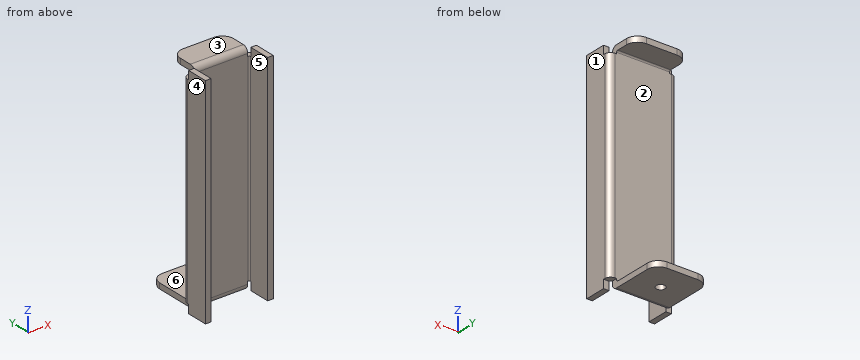
Autodesk Inventor part; units mm, degrees
ref_plane "YZ Plane" through (0, 0, 0) normal (1, 0, 0) x (0, 1, 0)
ref_plane "XZ Plane" through (0, 0, 0) normal (0, 1, 0) x (-1, 0, 0)
ref_plane "XY Plane" through (0, 0, 0) normal (0, 0, 1) x (1, 0, 0)
sketch "Эскиз1" plane through (0, 0, 0) normal (0, 0, 1) x (1, 0, 0)
  line L0 (0, 0) -> (0, 11.2754) construction
  line L1 (0, 0) -> (-17.0842, 0) construction
  line L2 (-12.15, 0) -> (12.15, 0)
  line L3 (12.15, 0) -> (12.15, 10.3)
  line L4 (12.15, 10.3) -> (-12.15, 10.3)
  line L5 (-12.15, 10.3) -> (-12.15, 0)
  line L6 (-10.15, 0) -> (10.15, 0)
  line L7 (10.15, 0) -> (10.15, 8.3)
  line L8 (10.15, 8.3) -> (-10.15, 8.3)
  line L9 (-10.15, 8.3) -> (-10.15, 0)
  dimension "d0" = 2
  dimension "d1" = 2
  dimension "d2" = 2
  dimension "d3" = 24.3
  dimension "d4" = 10.3
extrude "Выдавливание1" add sketch "Эскиз1" along normal mid plane 78 contours L5 L4 L3 L2 L7 L8 L9
sketch "Эскиз2" plane through (-12.15, 10.3, -39) normal (0, 1, 0) x (1, 0, 0)
  line L0 (0, 0) -> (24.3, 0)
  line L1 (2.65, 0) -> (21.65, 0)
  line L2 (21.65, 0) -> (21.65, -2)
  line L3 (21.65, -2) -> (2.65, -2)
  line L4 (2.65, -2) -> (2.65, 0)
  line L5 (24.3, -78) -> (0, -78)
  line L6 (2.65, -78) -> (21.65, -78)
  line L7 (21.65, -78) -> (21.65, -76)
  line L8 (21.65, -76) -> (2.65, -76)
  line L9 (2.65, -76) -> (2.65, -78)
  line L10 (12.15, -39) -> (12.15, -67.9082) construction
  dimension "d7" = 2
  dimension "d8" = 2
  dimension "d9" = 19
  dimension "d10" = 19
extrude "Выдавливание2" add sketch "Эскиз2" along normal blind 8.5 contours L5 L9 L8 L7
extrude "Выдавливание3" add sketch "Эскиз2" along normal blind 18 contours L0 L2 L3 L4
fillet "Сопряжение1" radius 4 4 edges at (9.5, 28.3, -38) (-9.5, 28.3, -38) (-9.5, 18.8, 38) (9.5, 18.8, 38)
sketch "Эскиз3" plane through (-9.5, 10.3, -37) normal (0, 0, 1) x (1, 0, 0)
  line L0 (9.5, -10.3) -> (9.5, 21.9843) construction
  circle A0 centre (9.5, 8) radius 1.6
  line L1 (15, 18) -> (4, 18)
  dimension "d16" = 3.2
  dimension "d17" = 10
extrude "Выдавливание4" cut sketch "Эскиз3" against normal blind 18
sketch "Эскиз4" plane through (0, 0, 39) normal (0, 0, 1) x (1, 0, 0)
  line L0 (12.15, 0) -> (12.15, 10.3)
  line L1 (9.5, 10.3) -> (12.15, 10.3)
  line L2 (12.15, 10.3) -> (12.15, 7.7)
  line L3 (12.15, 7.7) -> (9.5, 7.7)
  line L4 (9.5, 7.7) -> (9.5, 10.3)
  line L5 (10.15, 0) -> (12.15, 0)
  line L6 (-12.15, 10.3) -> (-9.5, 10.3)
  line L7 (-9.5, 10.3) -> (-15.4416, 10.3)
  line L8 (-15.4416, 10.3) -> (-15.4416, 7.7)
  line L9 (-15.4416, 7.7) -> (-9.5, 7.7)
  line L10 (-9.5, 7.7) -> (-9.5, 10.3)
  line L11 (-12.15, 0) -> (-10.15, 0)
  point P0 (0, 0)
  dimension "d20" = 7.7
  dimension "d21" = 7.7
extrude "Выдавливание5" cut sketch "Эскиз4" against normal blind 3
mirror "Зеркальное отражение1" about plane through (0, 0, 0) normal (0, 0, 1) of "Выдавливание5"
fillet "Сопряжение2" radius 2 4 edges at (0, 8.3, 39) (12.15, 10.3, 0) (-12.15, 10.3, 0) (0, 8.3, -39)
fillet "Сопряжение3" radius 0.5 4 edges at (0, 10.3, -37) (0, 10.3, 37) (10.15, 8.3, 0) (-10.15, 8.3, 0)
properties part number "крепление бабины"
CAD build for the part. Positions are in the model's coordinates, mm. Face numbers are marked on the shaded views. A direction names the side the tool comes from. Give positions to 0.01 mm unless a question says otherwise; leave off trailing zeros. Write each loop counter-clockwise with the first axis right and the second up, starting at its lowest first coordinate (ties: lowest second). Pieces come first, ordered by that corner, then holes. Notation, with made-up numbers: (-37, -12.75) -> (-16, -12.75) arc R17 cw to (-16, 11.25) -> close; hole circle Ø1 at (71.25, 43.25). An arc over 180 degrees is marked (long way). Return JSON: item names as keys, results as strings.
Item 1: Band-saw the part on B-B (x = 0). List the corners of the cut face in (y, z), then the cut area to 3 significant figures.
Answer below:
{"outline": "(8.3, -37) arc R2 ccw to (10.3, -39) -> (16.7, -39) -> (16.7, -37) -> (10.8, -37) arc R0.5 cw to (10.3, -36.5) -> (10.3, 36.5) arc R0.5 cw to (10.8, 37) -> (18.8, 37) -> (18.8, 39) -> (10.3, 39) arc R2 ccw to (8.3, 37) -> close; (19.9, -39) -> (28.3, -39) -> (28.3, -37) -> (19.9, -37) -> close", "area": "201 mm2"}
Item 2: Drop flat-ended pins along their axis: pin 1 (8 mm diameter, centred on x = -5, z = 15, fed in from -Y); pin 2 (1.6 mm diameter, centred on x = 11.5, z = 38, fed in from +Y); pin 3 (12 mm diameter, centred on y = 12.5, z = -19, fed in from -X); pin 4 (1.5 mm diameter, centred on y = 10, z = 37, fed in from -X). Give the stop position or say it passes through.
Answer below:
{"pin 1": "stops at y = 8.3", "pin 2": "stops at y = 7.7", "pin 3": "stops at x = -12.15", "pin 4": "stops at x = -9.5"}
Item 3: Tool access for the marked faces 4, 5 and 6: list every direction of +Z, -Z, +X, -X, +Y, -Y with a clear straight run to the whole face (end or side of a thin tool).
Answer below:
{"face 4": "+Z, -Z, -X, +Y, -Y", "face 5": "+Z, -Z, -Y", "face 6": "+X, -X, +Y"}
Item 4: Band-saw the part on A-A (y = 13.5). List the corners of the cut face in (x, z), then the cut area to 3 significant figures.
Answer below:
{"outline": "(-9.5, -39) -> (9.5, -39) -> (9.5, -37) -> (-9.5, -37) -> close; (-9.5, 37) -> (9.5, 37) -> (9.5, 39) -> (-9.5, 39) -> close", "area": "76.0 mm2"}
Item 5: Two-plate mould, pull along Z, no slides. Class the marked faces 1, 2 and 3: +Z half, -Z half, draft (parallel to the pull), parting line (faces both ways), or undercut.
Answer below:
{"face 1": "draft", "face 2": "undercut", "face 3": "+Z half"}
Item 6: Drill centre lines: probe 1 along X at (y, z) = (3, -26); probe 2 along Z at (x, y) = (-2, 14.75); probe 3 along Z at (x, y) = (-5.5, 24.5). Where is each one in solid material? Low to high.
Answer below:
{"probe 1": "x = -12.15 to -10.15, 10.15 to 12.15", "probe 2": "z = -39 to -37, 37 to 39", "probe 3": "z = -39 to -37"}
Item 7: Band-saw the part on D-D (y = 9.25). List the corners of the cut face in (x, z).
Answer below:
{"outline": "(-11.91, -36) -> (-9.5, -36) -> (-9.5, -38.7) -> (9.5, -38.7) -> (9.5, -36) -> (11.91, -36) -> (11.91, 36) -> (9.5, 36) -> (9.5, 38.7) -> (-9.5, 38.7) -> (-9.5, 36) -> (-11.91, 36) -> close"}
Item 8: Band-saw the part on C-C (z = -12). List the corners of the cut face in (x, y), then the cut area to 3 significant figures.
Answer below:
{"outline": "(-12.15, 0) -> (-10.15, 0) -> (-10.15, 7.8) arc R0.5 cw to (-9.65, 8.3) -> (9.65, 8.3) arc R0.5 cw to (10.15, 7.8) -> (10.15, 0) -> (12.15, 0) -> (12.15, 8.3) arc R2 ccw to (10.15, 10.3) -> (-10.15, 10.3) arc R2 ccw to (-12.15, 8.3) -> close", "area": "80.2 mm2"}
